Work out the finished part from the listing and answer in its coordinate system (mm). A direction names the side the tool comes from. Give positions to 0.01 mm unless a question says otherwise; leave off trailing zeros. Write each loop counter-clockwise with the first axis right and the second up, starting at its lowest first coordinate (ties: lowest second). Pieces come first, ordered by that corner, then holes.
1) A tool of negligible diameter and unlimited length cuts with its end or side. For faces 1 (the face through (-20, 14, 0)), 2 (the face through (-3, 14, 0)), 3 (the face through (-12, 22, 16)), from which of +Z, -Z, +X, -X, +Y, -Y can it reach the whole face along a straight path? Write none if from no direction.
2) Find section C-C (x = -14.75). Determine the outline of the cut face in (y, z).
3) Find section A-A (z = -31.5). Determine the outline of the cut face in (x, y).
4) Straight lines are drawn through the part: probe 1 along X at (y, z) = (13.25, -26); probe 2 along X at (y, z) = (4, 11.5); probe 3 along Z at (x, y) = (-6.75, 20.75). For each, find the intervals that lie inside material, in ascending order.
5) Find section D-D (z = -25). Determine the outline of the cut face in (x, y).
6) Determine the mould class of faces 4 (the face through (-14.5, 19, -17.8)), 5 (the face through (-12, 6, 16)), 6 (the face through (-12, 23, -14)) for opening direction Y: pulls with the +Y half, pulls with the -Y half, needs draft (parallel to the pull), parting line crosses it, or undercut.
7) Given pin 1 Ø6.5 at (y, z) = (20.5, 11.5) entering from +X; pin 2 Ø12 at (x, y) = (-10, 16.5) entering from +Z; pin 3 Ø11 at (x, z) = (-13.5, 15.5) entering from -Y; pin 4 Ø2.5 at (x, y) = (-7, 6) entering from -Z, each flat-ended and moving along its own axis, determine where each tip first touches the part or whether it passes through.
Autodesk Inventor part; units mm, degrees
ref_plane "YZ Plane" through (0, 0, 0) normal (1, 0, 0) x (0, 1, 0)
ref_plane "XZ Plane" through (0, 0, 0) normal (0, 1, 0) x (-1, 0, 0)
ref_plane "XY Plane" through (0, 0, 0) normal (0, 0, 1) x (1, 0, 0)
sketch "Szkic1" plane through (0, 0, 0) normal (0, 1, 0) x (-1, 0, 0)
  line L0 (0, 0) -> (24, 0)
  line L1 (24, 0) -> (24, -14)
  line L2 (24, -14) -> (0, -14)
  line L3 (0, -14) -> (0, 0)
  line L4 (17, 0) -> (7, 0)
  line L5 (7, 0) -> (7, 24)
  line L6 (7, 24) -> (17, 24)
  line L7 (17, 24) -> (17, 0)
  point P0 (7, 0)
  dimension "d0" = 24
  dimension "d1" = 14
  dimension "d2" = 10
  dimension "d3" = 24
  dimension "d4" = 7
extrude "Wyciągnięcie proste1" add sketch "Szkic1" along normal blind 28
fillet "Zaokrąglenie1" radius 14 2 edges at (-12, 28, 24) (-12, 0, 24)
sketch "Szkic2" plane through (-7, 0, 0) normal (1, 0, 0) x (0, 0, -1)
  circle A0 centre (-10, 14) radius 8
  line L0 (-10, 0) -> (0, 0)
  line L1 (-10, 22) -> (-24, 22)
  line L2 (-24, 22) -> (-24, 6)
  line L3 (-24, 6) -> (-10, 6)
  line L4 (-10, 6) -> (-10, 22)
  dimension "d8" = 16
  dimension "d9" = 14
extrude "Wyciągnięcie proste2" cut sketch "Szkic2" against normal through all
sketch "Szkic3" plane through (0, 0, -14) normal (0, 0, -1) x (-1, 0, 0)
  line L0 (0, 0) -> (0, 28)
  line L1 (24, 0) -> (24, 28)
  line L2 (0, 19) -> (24, 19)
  line L3 (24, 19) -> (24, 9)
  line L4 (24, 9) -> (0, 9)
  line L5 (0, 9) -> (0, 19)
  line L6 (0, 28) -> (24, 28)
  line L7 (0, 0) -> (24, 0)
  point P0 (0, 9)
  dimension "d12" = 9
  dimension "d13" = 9
extrude "Wyciągnięcie proste3" add sketch "Szkic3" along normal blind 24 contours L0 L2 L1 L4
full round fillet "Zaokrąglenie pełne1" first side at (0, 12.3333, -4.6667) centre faces at (-8, 15.6667, -38) second side at (-24, 12.3333, -4.6667)
sketch "Szkic4" plane through (-24, 19, -14) normal (0, 1, 0) x (1, 0, 0)
  arc A0 (24, 12) -> (0, 12) centre (12, 12) ccw
  point P0 (24, -14)
hole "Otwór1" at (-12, 19, -26) direction (0, -1, 0) diameter 16.5 end through all
Results:
1. face 1: +Z, -X, +Y, -Y
1. face 2: +Z, +X, +Y, -Y
1. face 3: +Z, +X, -X
2. outline: (0, -14) - (9, -14) - (9, -18.22) - (19, -18.22) - (19, -14) - (28, -14) - (28, 10) arc R14 ccw to (22, 21.49) - (22, 10) arc R8 cw to (6, 10) - (6, 21.49) arc R14 ccw to (0, 10) - close; (9, -37.68) - (19, -37.68) - (19, -33.78) - (9, -33.78) - close
3. outline: (-22.67, 9) - (-18.15, 9) - (-18.15, 19) - (-22.67, 19) - close; (-5.85, 9) - (-1.33, 9) - (-1.33, 19) - (-5.85, 19) - close
4. probe 1: x = -24 to -20.25, -3.75 to 0
4. probe 2: x = -17 to -7
4. probe 3: z = -14 to 0
5. outline: (-24, 9) - (-20.19, 9) - (-20.19, 19) - (-24, 19) - close; (-3.81, 9) - (0, 9) - (0, 19) - (-3.81, 19) - close
6. face 4: pulls with the +Y half
6. face 5: undercut
6. face 6: needs draft
7. pin 1: stops at x = -7
7. pin 2: stops at z = 21.49
7. pin 3: stops at y = 0
7. pin 4: stops at z = -14
